The figure shows three views and two pictorial views of one solid part (mm, origin at its lowest corner). Answer the questions. Give positions to 0.01 mm unless a question says otherwise; leave off trailing zeros. Loops run counter-clockwise (first coordinate to the right, second up) from the corner with the lowest first, then second, coordinate; pieces in that order, holes last. Notation, with made-up numbers: M -5,46 L 49,46 A25 ccw 49,62 Z; hole C 28.25,-21.5 d3. An arc over 180 degrees is marked long. Answer as a JSON object with one key per item and string values. Group by question number.
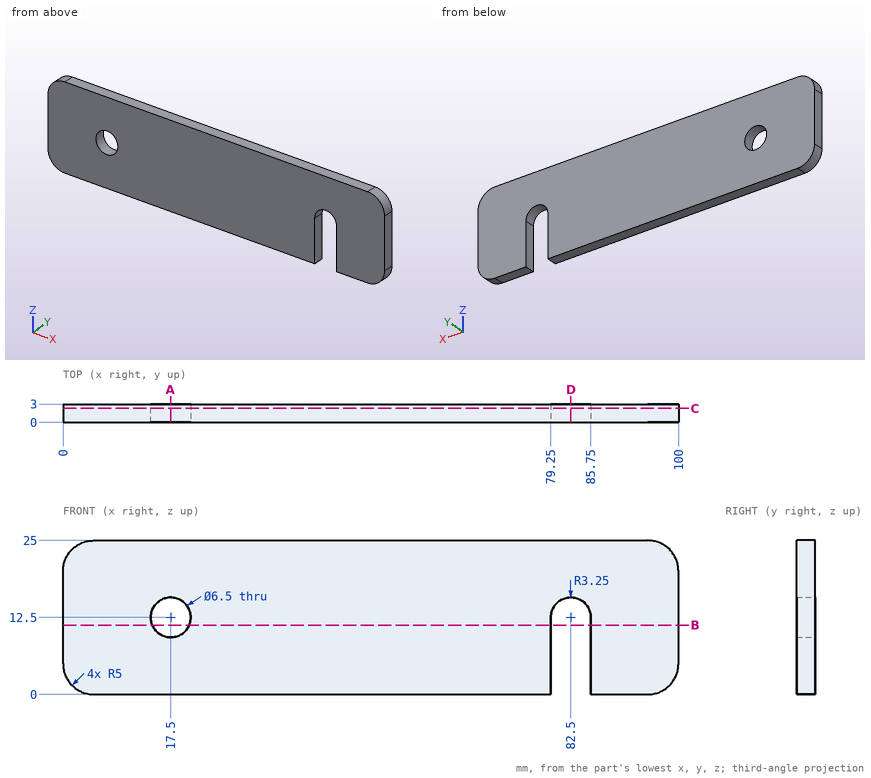
Item 1: A cutting plane is placed at B-B (z = 11.25). Determine the outline of the cut face in (x, y).
Item 2: A cutting plane is placed at C-C (y = 2.3). Determine the outline of the cut face in (x, z).
Item 3: A cutting plane is placed at D-D (x = 82.5). Determine the outline of the cut face in (y, z).
Item 4: Find the intervals of material crossed by probe 1 along X at (y, z) = (2.25, 12.5); probe 2 along Z at (x, y) = (17.5, 1.8); probe 3 along X at (y, z) = (2.1, 14.25), in increasing order. Write a range as [from, to].
Item 5: A cutting plane is placed at A-A (x = 17.5). Determine the outline of the cut face in (y, z).
Item 6: Given pin 1 Ø10 at (x, z) = (84, 16.5) entering from -Y; pin 2 Ø5 at (x, z) = (17.5, 12.5) entering from -Y, each flat-ended and moving along its own axis, determine where each tip first touches the part or whether it passes through.
The answers:
{
 "1": {"outline": "M 0,0 L 14.5,0 L 14.5,3 L 0,3 Z; M 20.5,0 L 79.25,0 L 79.25,3 L 20.5,3 Z; M 85.75,0 L 100,0 L 100,3 L 85.75,3 Z"},
 "2": {"outline": "M 0,5 A5 ccw 5,0 L 79.25,0 L 79.25,12.5 A3.25 cw 85.75,12.5 L 85.75,0 L 95,0 A5 ccw 100,5 L 100,20 A5 ccw 95,25 L 5,25 A5 ccw 0,20 Z; hole C 17.5,12.5 d6.5"},
 "3": {"outline": "M 0,15.75 L 3,15.75 L 3,25 L 0,25 Z"},
 "4": {"probe 1": "x = [0, 14.25], [20.75, 79.25], [85.75, 100]", "probe 2": "z = [0, 9.25], [15.75, 25]", "probe 3": "x = [0, 14.76], [20.24, 79.76], [85.24, 100]"},
 "5": {"outline": "M 0,0 L 3,0 L 3,9.25 L 0,9.25 Z; M 0,15.75 L 3,15.75 L 3,25 L 0,25 Z"},
 "6": {"pin 1": "stops at y = 0", "pin 2": "passes through"}
}
